from build123d import *

# Parameters (mm, degrees)
DODANIE_WYCI_GNI_CIE1_DEPTH = 2
SZKIC2_R                    = 0.6
SZKIC2_R_2                  = 8
WYTNIJ_WYCI_GNI_CIE1_DEPTH  = 2


with BuildPart() as part:
    # Szkic1 → Dodanie-wyciągnięcie1 (new body)
    with BuildSketch(Plane.XY):
        Polygon((-111, 8.2), (188, 8.2), (188, -8.2), (31, -8.2), (31, -9.7), (-31, -9.7), (-31, -8.2), (-111, -8.2), (-121, -8.2), (-121, 8.2), align=None)
    extrude(amount=DODANIE_WYCI_GNI_CIE1_DEPTH)

    # Szkic2 → Wytnij-wyciągnięcie1 (cut)
    with BuildSketch(Plane(origin=(0, 0, 0), x_dir=(-1, 0, 0), z_dir=(0, 0, -1))):
        with Locations((-186.5, -6.7)):
            Circle(SZKIC2_R)
        with Locations((-186.5, 11.2)):
            Circle(SZKIC2_R)
        with Locations((186.5, 11.2)):
            Circle(SZKIC2_R)
        with Locations((186.5, -11.2)):
            Circle(SZKIC2_R)
        with Locations((-148.220730504, -8.2)):
            Circle(SZKIC2_R_2)
    extrude(amount=-WYTNIJ_WYCI_GNI_CIE1_DEPTH, mode=Mode.SUBTRACT)


solid = part.part
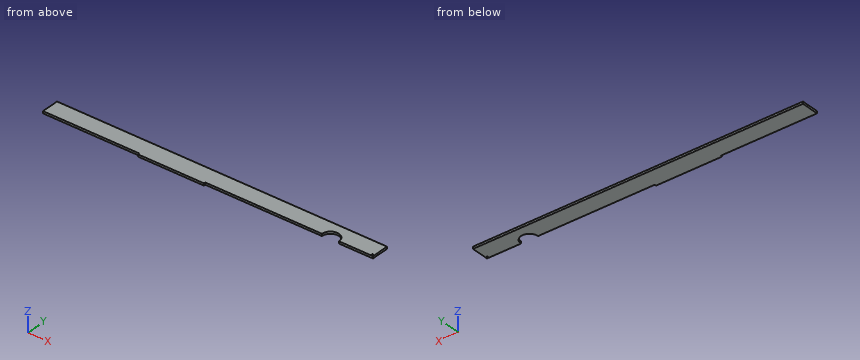
Here's how the part is built. I have some questions about the finished solid (model axes, mm). Give positions to 0.01 mm unless a question says otherwise; leave off trailing zeros. Loops run counter-clockwise (first coordinate to the right, second up) from the corner with the lowest first, then second, coordinate; pieces in that order, holes last. Notation, with made-up numbers: (-39.75, 1.25) -> (-1.75, 1.25) arc R18 ccw to (-1.75, 23.25) -> close; hole circle Ø8 at (-20, 18.25). An arc over 180 degrees is marked (long way). Answer as a JSON object with one key per item and string values. Group by question number.
Item 1: I need wall thicknesses on L1, parallel to X at y = -7, z = 0.95; L2, parallel to Y at x = 186.5, z = 0.55; L3, parallel to X at y = -2.5, z = 1.05. Which ranges of each line are inside material? Lowest first, please.
Item 2: Imagine slicing it at B-B on x = 93. Write out the boundary of the cut face in (y, z).
Item 3: Imagine slicing it at A-A on z = 1.25. Write out the boundary of the cut face in (x, y), then the cut area to 3 significant figures.
Item 4: Will these pins go through, and if not, where does the flat tip stop? pin 1 (1 mm diameter, centred on x = 71.5, z = 1.5, fed in from -Y); pin 2 (0.8 mm diameter, centred on y = -9, z = 1.5, fed in from -X).
Answer list:
{
 "1": {"L1": "x = -121 to 140.31, 156.13 to 185.98, 187.02 to 188", "L2": "y = -8.2 to -7.3, -6.1 to 8.2", "L3": "x = -121 to 142.61, 153.83 to 188"},
 "2": {"outline": "(-8.2, 0) -> (8.2, 0) -> (8.2, 2) -> (-8.2, 2) -> close"},
 "3": {"outline": "(-121, -8.2) -> (-31, -8.2) -> (-31, -9.7) -> (31, -9.7) -> (31, -8.2) -> (140.22, -8.2) arc R8 cw to (156.22, -8.2) -> (188, -8.2) -> (188, 8.2) -> (-121, 8.2) -> close; hole circle Ø1.2 at (186.5, -6.7)", "area": "5,060 mm2"},
 "4": {"pin 1": "stops at y = -8.2", "pin 2": "stops at x = -31"}
}
